Work out the finished part from the listing and answer in its coordinate system (mm). Face numbers are marked on the shaded views. A direction names the side the tool comes from. Round coordinates to 2 decimals unless told otherwise and drop trailing zeros. Write each loop counter-clockwise with the first axis right and the second up, starting at its lowest first coordinate (ties: lowest second). Pieces come first, ordered by that corner, then holes. Notation, with made-up numbers: (69, 28) - (87, 28) arc R12 ccw to (87, 40) - close; hole circle Ø1 at (80, -7.75). An arc over 180 degrees is marked (long way). Answer as a JSON object with one key per item and string values.
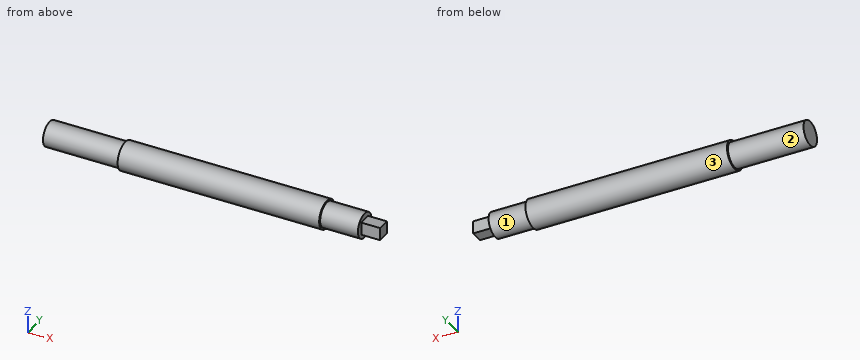
```python
from build123d import *

# Parameters (mm, degrees)
F0_R          = 14.2875
F0_R_2        = 12.4968
F1_DEPTH      = 101.6
F1_DEPTH_BACK = 101.6
F0_W          = 12.7
F0_H          = 12.7
F2_DEPTH      = 139.7
F2_DEPTH_BACK = 177.8
F3_DEPTH      = 158.75
F3_DEPTH_BACK = 177.8


with BuildPart() as f1:
    # F0 (on Right) → F1 (new body, two sides)
    with BuildSketch(Plane.YZ) as f1_sk:
        Circle(F0_R)
        Circle(F0_R_2, mode=Mode.SUBTRACT)
    extrude(amount=F1_DEPTH)
    extrude(f1_sk.sketch, amount=-F1_DEPTH_BACK)

    # F0 (on Right) → F2 (join, two sides)
    with BuildSketch(Plane.YZ) as f2_sk:
        Circle(F0_R_2)
        Rectangle(F0_W, F0_H, mode=Mode.SUBTRACT)
    extrude(amount=F2_DEPTH)
    extrude(f2_sk.sketch, amount=-F2_DEPTH_BACK)

    # F0 (on Right) → F3 (join, two sides)
    with BuildSketch(Plane.YZ) as f3_sk:
        Rectangle(F0_W, F0_H)
    extrude(amount=F3_DEPTH)
    extrude(f3_sk.sketch, amount=-F3_DEPTH_BACK)


solid = f1.part
```
Item 1: For the marked faces 1, 2 and 3, determine the directions among +Z, -Z, +X, -X, +Y, -Y from which every point of the face is accessible in a straight line to the end or side of a thin tool.
Results found:
{"face 1": "+X", "face 2": "-X", "face 3": "+X, -X"}
Item 2: Consider line 1 along X through (y, z) = (-8.75, -4.5); line 2 along Z through (x, y) = (39, 1); line 3 along X through (y, z) = (-11, 6). Determine where each line is inside the solid, lowest interval first.
Results found:
{"line 1": "-177.8 to 139.7", "line 2": "-14.25 to 14.25", "line 3": "-101.6 to 101.6"}
Item 3: A cutting plane is placed at C-C (x = 10). Write down the section's boundary in (y, z) (1 decimal), and give its area (3 significant figures).
Results found:
{"outline": "circle Ø28.6 at (0, 0)", "area": "641 mm²"}
Item 4: A cutting plane is placed at D-D (x = -139.5). Write down the section's boundary in (y, z), and give its area (3 significant figures).
Results found:
{"outline": "circle Ø24.99 at (0, 0)", "area": "491 mm²"}
Item 5: A cutting plane is placed at A-A (z = 0). Write down the section's boundary in (x, y), and give its area (3 significant figures).
Results found:
{"outline": "(-177.8, -12.5) - (-101.6, -12.5) - (-101.6, -14.29) - (101.6, -14.29) - (101.6, -12.5) - (139.7, -12.5) - (139.7, -6.35) - (158.75, -6.35) - (158.75, 6.35) - (139.7, 6.35) - (139.7, 12.5) - (101.6, 12.5) - (101.6, 14.29) - (-101.6, 14.29) - (-101.6, 12.5) - (-177.8, 12.5) - close", "area": "8,910 mm²"}
Item 6: Each of these flat-tipped pins is pushed along its axis until it touches: P1, Ø6, axis at x = -135.5, z = -8, coming from the -Y side; P2, Ø1.5, axis at x = 34, y = -5.5, coming from the -Z side; P3, Ø1.5, axis at x = -128.5, z = -1, coming from the -Y side; P4, Ø2, axis at x = 66, z = 1, coming from the -Y side. Where does it stop, or does it pass through?
Results found:
{"P1": "y = -11.45", "P2": "z = -13.47", "P3": "y = -12.49", "P4": "y = -14.29"}
